The model under review builds one solid part; all positions refer to its coordinate system, in mm. A direction names the side the tool comes from. Round coordinates to 2 decimals unless told otherwise and drop trailing zeros. Write each loop counter-clockwise with the first axis right and the second up, starting at its lowest first coordinate (ties: lowest second). Pieces come first, ordered by that corner, then holes. Notation, with made-up numbers: (55, 64.25) -> (71, 64.25) arc R23 ccw to (71, 95.25) -> close; hole circle Ø7 at (27.5, -24.5). An arc over 180 degrees is marked (long way). Return JSON: item names as keys, results as strings. Group by question number.
1. Take a section at D-D, the plane x = 198. Write out the cut boundary in (y, z).
2. Mouldability with a two-part tool opening along Z and no side actions: class faces 1 (the flat face through (205, 54, 7)), 2 (the flat face through (135, 28, 220)), 3 (the cylindrical face through (2, 53, 1)) as pulls with the +Z half, pulls with the -Z half, needs draft (parallel to the pull), parting line crosses it, or undercut.
3. For line 1 along X through (y, z) = (92.5, 108); line 2 along X through (y, z) = (95, 218), list the stretches that pass through material, from the lowest coordinate up. Write a range as from..to.
4. Take a section at B-B, the plane x = 110. Write out the cut boundary in (y, z), then the cut area to 3 significant figures.
5. Take a section at C-C, the plane z = 162. Write out the cut boundary in (x, y), then the cut area to 3 significant figures.
6. Tool access review of faces 4 (the cylindrical face through (86, 37, 3)), 5 (the cylindrical face through (14, 56, 207)): name each direction out of +Z, -Z, +X, -X, +Y, -Y from which nothing blocks a thin tool from reaching the whole face with its end or side.
7. Clearance check with flat-ended pins moving along their axes: P1, Ø1.8, axis at x = 212, z = 212.5, coming from the +Y side; P2, Ø1, axis at x = 213, z = 6.5, coming from the +Y side; P3, Ø4, axis at x = 176.5, z = 101.5, coming from the +Y side. State where each tip first meets the part, or that it passes through.
Autodesk Fusion 360 part; units mm, degrees
sketch "Sketch1" plane through (0, 0, 0) normal (0, 1, 0) x (1, 0, 0)
  line L0 (0, 0) -> (220, 0)
  line L1 (220, 0) -> (220, -220)
  line L2 (220, -220) -> (0, -220)
  line L3 (0, -220) -> (0, 0)
  dimension "d1" = 220
  dimension "d2" = 220
extrude "Extrude1" add sketch "Sketch1" along normal blind 5
sketch "Sketch2" plane through (0, 5, 0) normal (0, 1, 0) x (-1, 0, 0)
  line L0 (0, 220) -> (-220, 220)
  line L1 (-220, 220) -> (-220, 0)
  line L2 (-220, 0) -> (0, 0)
  line L3 (0, 0) -> (0, 220)
  line L4 (0, 0) -> (-10, 0)
  line L5 (-10, 220) -> (0, 220)
  line L6 (0, 220) -> (0, 0)
  line L7 (0, 0) -> (-5, 0)
  line L8 (-5, 0) -> (-5, 220)
  line L9 (-5, 220) -> (0, 220)
  line L10 (0, 220) -> (0, 0)
  line L11 (0, 0) -> (-220, 0)
  line L12 (-220, 0) -> (-220, 5)
  line L13 (-220, 5) -> (0, 5)
  line L14 (0, 5) -> (0, 0)
  line L15 (0, 220) -> (-220, 220)
  line L16 (-220, 220) -> (-220, 215)
  line L17 (-220, 215) -> (0, 215)
  line L18 (0, 215) -> (0, 220)
  line L19 (-220, 220) -> (-215, 220)
  line L20 (-215, 220) -> (-215, 0)
  line L21 (-215, 0) -> (-220, 0)
  line L22 (-220, 0) -> (-220, 220)
  dimension "d5" = 5
  dimension "d6" = 5
extrude "Extrude2" add sketch "Sketch2" along normal blind 100 contours L0 L3 L5 L6 L8 L9 L10 L15 L17 L18 | L0 L5 L8 L15 L17 L20 | L3 L6 L8 L10 L13 L17 | L2 L3 L4 L6 L7 L8 L10 L11 L13 L14 | L0 L1 L15 L16 L17 L19 L20 L22 | L2 L4 L8 L11 L13 L20 | L1 L13 L17 L20 L22 | L1 L2 L11 L12 L13 L20 L21 L22
sketch "Sketch3" plane through (0, 0, 5) normal (0, 0, 1) x (1, 0, 0)
  line L0 (5, 5) -> (215, 5)
  line L1 (215, 5) -> (215, 105)
  line L2 (215, 105) -> (5, 105)
  line L3 (5, 105) -> (5, 5)
sketch "Sketch4" plane through (0, 5, 0) normal (0, 1, 0) x (-1, 0, 0)
  line L0 (-5, 5) -> (-5, 215)
  line L1 (-5, 215) -> (-215, 215)
  line L2 (-215, 215) -> (-215, 5)
  line L3 (-215, 5) -> (-5, 5)
  line L4 (-5, 5) -> (-15, 5)
  line L5 (-15, 5) -> (-15, 15)
  line L6 (-15, 15) -> (-5, 15)
  line L7 (-5, 15) -> (-5, 5)
  line L8 (-215, 5) -> (-205, 5)
  line L9 (-205, 5) -> (-205, 15)
  line L10 (-205, 15) -> (-215, 15)
  line L11 (-215, 15) -> (-215, 5)
  line L12 (-5, 215) -> (-15, 215)
  line L13 (-15, 215) -> (-15, 205)
  line L14 (-15, 205) -> (-5, 205)
  line L15 (-5, 205) -> (-5, 215)
  line L16 (-215, 215) -> (-205, 215)
  line L17 (-205, 215) -> (-205, 205)
  line L18 (-205, 205) -> (-215, 205)
  line L19 (-215, 205) -> (-215, 215)
  dimension "d10" = 10
  dimension "d11" = 10
  dimension "d12" = 10
  dimension "d13" = 10
  dimension "d14" = 10
  dimension "d15" = 10
  dimension "d16" = 10
  dimension "d17" = 10
extrude "Extrude3" add sketch "Sketch4" along normal blind 100 contours L0 L3 L4 L5 L6 L7 | L0 L1 L12 L13 L14 L15 | L2 L3 L8 L9 L10 L11 | L1 L2 L16 L17 L18 L19
fillet "Fillet1" radius 5 4 edges at (205, 55, 15) (15, 55, 15) (15, 55, 205) (205, 55, 205)
sketch "Sketch5" plane through (0, 0, 220) normal (0, 0, 1) x (1, 0, 0)
  line L0 (0, 0) -> (220, 0)
  line L1 (220, 0) -> (220, 105)
  line L2 (220, 105) -> (0, 105)
  line L3 (0, 105) -> (0, 0)
  line L4 (0, 0) -> (110, 0)
  line L5 (110, 0) -> (110, 55)
  line L6 (110, 55) -> (150, 55)
  line L7 (150, 55) -> (150, 15)
  line L8 (150, 15) -> (110, 15)
  line L9 (110, 15) -> (110, 55)
  line L10 (150, 15) -> (70, 15)
  line L11 (70, 15) -> (70, 95)
  line L12 (70, 95) -> (150, 95)
  line L13 (150, 95) -> (150, 15)
  circle A0 centre (110, 55) radius 30
  dimension "d22" = 55
  dimension "d23" = 40
  dimension "d24" = 40
  dimension "d25" = 80
  dimension "d26" = 80
  dimension "d27" = 60
extrude "Extrude4" cut sketch "Sketch5" against normal blind 270 contours L5 L6 L9 A0 | L5 L6 L9 A0
hole "Hole1" at (70, 95, 220) at (150, 95, 220) at (70, 15, 220) at (150, 15, 220) direction (0, 0, -1) diameter 3.5 depth 10000 tip angle 118
sketch "Sketch6" plane through (0, 105, 0) normal (0, 1, 0) x (-1, 0, 0)
  arc A0 (-210, 205) -> (-205, 210) centre (-210, 210) ccw
  line L0 (-205, 210) -> (-205, 215)
  line L1 (-205, 215) -> (-15, 215)
  line L2 (-15, 215) -> (-15, 210)
  arc A1 (-15, 210) -> (-10, 205) centre (-10, 210) ccw
  line L3 (-10, 205) -> (-5, 205)
  line L4 (-5, 205) -> (-5, 15)
  line L5 (-5, 15) -> (-10, 15)
  arc A2 (-10, 15) -> (-15, 10) centre (-10, 10) ccw
  line L6 (-15, 10) -> (-15, 5)
  line L7 (-15, 5) -> (-205, 5)
  line L8 (-205, 5) -> (-205, 10)
  arc A3 (-205, 10) -> (-210, 15) centre (-210, 10) ccw
  line L9 (-210, 15) -> (-215, 15)
  line L10 (-215, 15) -> (-215, 205)
  line L11 (-215, 205) -> (-210, 205)
  line L12 (0, 0) -> (0, 220)
  line L13 (0, 220) -> (-220, 220)
  line L14 (-220, 220) -> (-220, 0)
  line L15 (-220, 0) -> (0, 0)
  line L16 (0, 0) -> (-7.0711, 7.0711)
  line L17 (0, 0) -> (10, 0) construction
  line L18 (-220, 0) -> (-212.9289, 7.0711)
  line L19 (-220, 0) -> (-210, 0) construction
  line L20 (0, 220) -> (-7.0711, 212.9289)
  line L21 (0, 220) -> (10, 220) construction
  line L22 (-220, 220) -> (-212.9289, 212.9289)
  line L23 (-220, 220) -> (-210, 220) construction
  dimension "d33" = 135
  dimension "d34" = 10
  dimension "d35" = 45
  dimension "d36" = 10
  dimension "d37" = 135
  dimension "d38" = 10
  dimension "d39" = 10
  dimension "d40" = 45
hole "Hole2" at (7.0711, 105, 212.9289) at (212.9289, 105, 212.9289) at (212.9289, 105, 7.0711) at (7.0711, 105, 7.0711) direction (0, -1, 0) diameter 4.7 depth 4.3 tip angle 180
hole "Hole3" at (7.0711, 105, 212.9289) at (212.9289, 105, 212.9289) at (212.9289, 105, 7.0711) at (7.0711, 105, 7.0711) direction (0, -1, 0) diameter 3.5 depth 8 tip angle 180
fillet "Fillet2" radius 5 4 edges at (220, 52.5, 220) (0, 52.5, 220) (0, 52.5, 0) (220, 52.5, 0)
Output:
{
 "1": {"outline": "(0, 0) -> (105, 0) -> (105, 5) -> (5, 5) -> (5, 215) -> (105, 215) -> (105, 220) -> (0, 220) -> close"},
 "2": {"face 1": "undercut", "face 2": "pulls with the +Z half", "face 3": "pulls with the -Z half"},
 "3": {"line 1": "x = 0..5, 215..220", "line 2": "x = 1..68.25, 71.75..148.25, 151.75..219"},
 "4": {"outline": "(0, 0) -> (25, 0) -> (25, 5) -> (5, 5) -> (5, 215) -> (25, 215) -> (25, 220) -> (0, 220) -> close; (85, 0) -> (105, 0) -> (105, 5) -> (85, 5) -> close; (85, 215) -> (105, 215) -> (105, 220) -> (85, 220) -> close", "area": "1,500 mm^2"},
 "5": {"outline": "(0, 0) -> (220, 0) -> (220, 105) -> (215, 105) -> (215, 5) -> (5, 5) -> (5, 105) -> (0, 105) -> close", "area": "2,100 mm^2"},
 "6": {"face 4": "+Z, -Z", "face 5": "+Y"},
 "7": {"P1": "stops at y = 100.7", "P2": "stops at y = 97", "P3": "stops at y = 5"}
}
